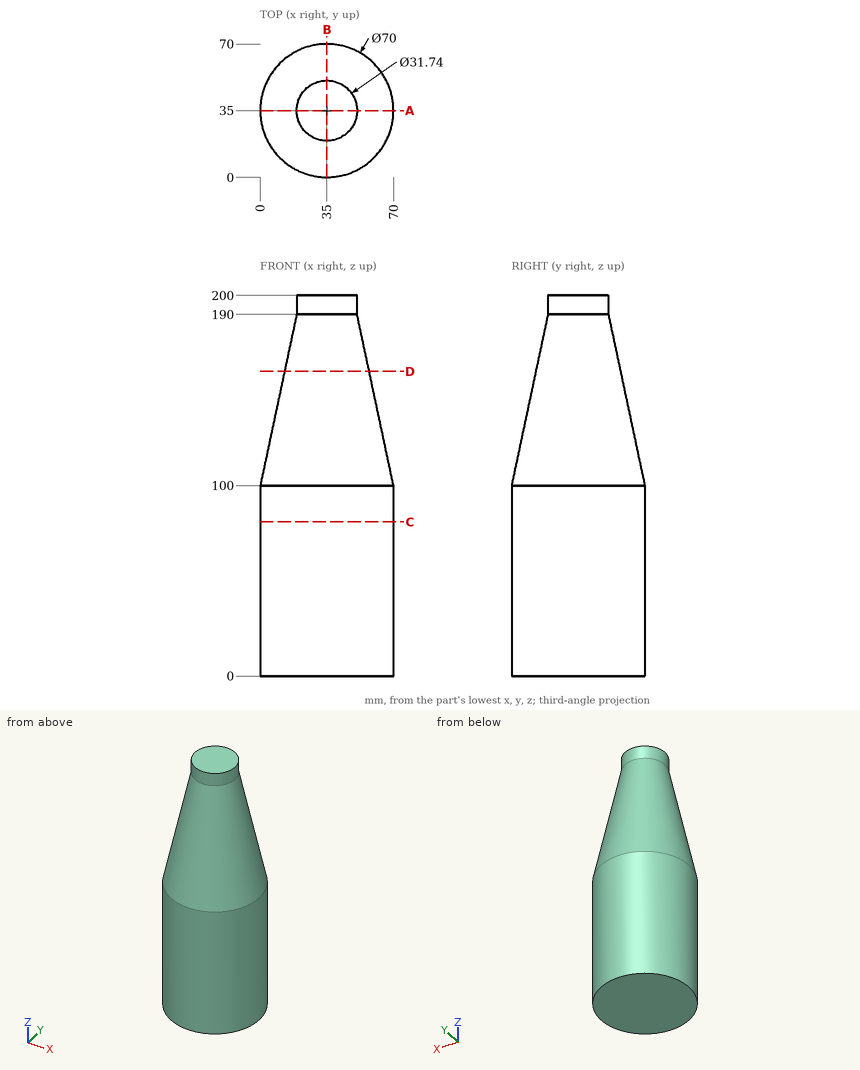
Study the drawing (mm; zero at the part's minimum x, y, z) and answer. Round coordinates to 2 decimals unless told otherwise and drop trailing zeros. Write each loop counter-clockwise with the first axis right and the second up, starting at its lowest first coordinate (ties: lowest second). Pieces come first, ordered by that corner, then holes. Notation, with made-up numbers: (12.25, 53.5) -> (59.25, 53.5) arc R32 ccw to (59.25, 89.5) -> close; hole circle Ø1 at (88, -22). An arc over 180 degrees is marked (long way). Answer as CSV lines item,"result". Start each with the question number.
(1) The part is cut by section C-C, the plane z = 81. Give the vertices of the cut face in (x, y), then the cut area to 3 significant figures.
(2) The part is cut by section A-A, the plane y = 35. Give the vertices of the cut face in (x, z).
(3) Each of these flat-tipped pins is pushed along its axis until it touches: pin 1 (5 mm diameter, centred on y = 16.5, z = 58, fed in from -X); pin 2 (4 mm diameter, centred on y = 15, z = 65, fed in from -X); pin 3 (4 mm diameter, centred on x = 55, z = 52.5, fed in from -Y). Where does it stop, or does it pass through?
(4) Find the intervals of material crossed by probe 1 along X at (y, z) = (36, 75.5); probe 2 along X at (y, z) = (48, 36); probe 3 along Y at (x, z) = (18, 37), in increasing order.
(5) The part is cut by section D-D, the plane z = 160. Give the vertices of the cut face in (x, y).
Output values:
1,outline,"circle Ø70 at (35, 35)"
1,area,"3,850 mm²"
2,outline,"(0, 0) -> (70, 0) -> (70, 100) -> (50.87, 190) -> (50.87, 200) -> (19.13, 200) -> (19.13, 190) -> (0, 100) -> close"
3,pin 1,"stops at x = 3.87"
3,pin 2,"stops at x = 4.98"
3,pin 3,"stops at y = 4.98"
4,probe 1,"x = 0.01 to 69.99"
4,probe 2,"x = 2.5 to 67.5"
4,probe 3,"y = 4.41 to 65.59"
5,outline,"circle Ø44.49 at (35, 35)"
